CAD build for the part. Positions are in the model's coordinates, mm. Face numbers are marked on the shaded views. A direction names the side the tool comes from. Coordinates: 2 decimals unless noted, no trailing zeros. Order: outer loops, then holes, each group sorted by start corner. A loop starts at its lowest first (then second) coordinate and runs counter-clockwise, first axis right, second up. Notation, with made-up numbers: M -13,89 L 30,89 A25 cw 30,116 Z; hole C -23,71.25 d2. An arc over 180 degrees is marked long. Write item = value, one per line.
from build123d import *

# Parameters (mm, degrees)
AUFSATZ_LINEAR_AUSTRAGEN1_DEPTH = 13
SKIZZE2_W                       = 16
SKIZZE2_H                       = 7
SCHNITT_LINEAR_AUSTRAGEN1_DEPTH = 10
SKIZZE4_R                       = 2.5
SCHNITT_LINEAR_AUSTRAGEN2_DEPTH = 3
SKIZZE5_R                       = 3.5
SKIZZE5_R_2                     = 2
SCHNITT_LINEAR_AUSTRAGEN3_DEPTH = 4
SKIZZE6_R                       = 2.1
SCHNITT_LINEAR_AUSTRAGEN4_DEPTH = 4
SKIZZE7_R                       = 5
SKIZZE7_R_2                     = 3.5
AUFSATZ_LINEAR_AUSTRAGEN2_DEPTH = 0.5
AUFSATZ_LINEAR_START            = 0.5
SKIZZE8_R                       = 5
SKIZZE8_R_2                     = 2.1
AUFSATZ_LINEAR_AUSTRAGEN3_DEPTH = 0.5


with BuildPart() as part:
    # Skizze1 → Aufsatz-Linear austragen1 (new body)
    with BuildSketch(Plane.XY):
        with BuildLine():
            ThreePointArc((5, 0), (3.535533906, 3.535533906), (0, 5))
            Line((0, 5), (0, 2))
            ThreePointArc((0, 2), (1.414213562, 1.414213562), (2, 0))
            ThreePointArc((2, 0), (1.414213562, -1.414213562), (0, -2))
            Line((0, -2), (0, -5))
            ThreePointArc((0, -5), (3.535533906, -3.535533906), (5, 0))
        make_face()
        with BuildLine():
            Line((0, 2), (0, 5))
            ThreePointArc((0, 5), (-5, 0), (0, -5))
            Line((0, -5), (0, -2))
            ThreePointArc((0, -2), (-2, 0), (0, 2))
        make_face()
        with BuildLine():
            Line((20, 5), (0, 5))
            ThreePointArc((0, 5), (3.535533906, 3.535533906), (5, 0))
            ThreePointArc((5, 0), (3.535533906, -3.535533906), (0, -5))
            Line((0, -5), (20, -5))
            Line((20, -5), (20, 5))
        make_face()
    extrude(amount=AUFSATZ_LINEAR_AUSTRAGEN1_DEPTH)

    # Skizze2 → Schnitt-Linear austragen1 (cut)
    with BuildSketch(Plane(origin=(0, 5, 0), x_dir=(1, 0, 0), z_dir=(0, 1, 0))):
        with Locations((12, -6.5)):
            Rectangle(SKIZZE2_W, SKIZZE2_H)
    extrude(amount=-SCHNITT_LINEAR_AUSTRAGEN1_DEPTH, mode=Mode.SUBTRACT)

    # Skizze4 → Schnitt-Linear austragen2 (cut)
    with BuildSketch(Plane.XY.offset(3)):
        with Locations((14, 0)):
            Circle(SKIZZE4_R)
    extrude(amount=-SCHNITT_LINEAR_AUSTRAGEN2_DEPTH, mode=Mode.SUBTRACT)

    # Skizze5 → Schnitt-Linear austragen3 (cut)
    with BuildSketch(Plane(origin=(0, 0, 0), x_dir=(-1, 0, 0), z_dir=(0, 0, -1))):
        Circle(SKIZZE5_R)
        Circle(SKIZZE5_R_2, mode=Mode.SUBTRACT)
    extrude(amount=-SCHNITT_LINEAR_AUSTRAGEN3_DEPTH, mode=Mode.SUBTRACT)

    # Skizze6 → Schnitt-Linear austragen4 (cut)
    with BuildSketch(Plane(origin=(0, 0, 10), x_dir=(-1, 0, 0), z_dir=(0, 0, -1))):
        with Locations((-14, 0)):
            Circle(SKIZZE6_R)
    extrude(amount=-SCHNITT_LINEAR_AUSTRAGEN4_DEPTH, mode=Mode.SUBTRACT)

    # Skizze7 → Aufsatz-Linear austragen2 (add)
    with BuildSketch(Plane.XY.offset(3)):
        with Locations(Location((14, 0, 0), (0, 0, 270))):
            Circle(SKIZZE7_R)
        with Locations((14, 0)):
            Circle(SKIZZE7_R_2, mode=Mode.SUBTRACT)
    extrude(amount=AUFSATZ_LINEAR_AUSTRAGEN2_DEPTH)

    # Skizze8 → Aufsatz-Linear austragen3 (add)
    with BuildSketch(Plane(origin=(0, 0, 10), x_dir=(-1, 0, 0), z_dir=(0, 0, -1)).offset(AUFSATZ_LINEAR_START)):
        with Locations(Location((-14, 0, 0), (0, 0, 270))):
            Circle(SKIZZE8_R)
        with Locations((-14, 0)):
            Circle(SKIZZE8_R_2, mode=Mode.SUBTRACT)
    extrude(amount=-AUFSATZ_LINEAR_AUSTRAGEN3_DEPTH)


solid = part.part
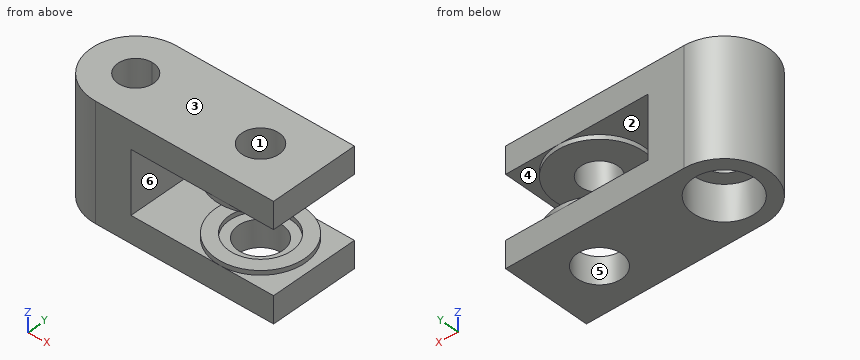
(1) Tool access for the marked faces 4, 5 and 6: list every direction of +Z, -Z, +X, -X, +Y, -Y with a clear straight run to the whole face (end or side of a thin tool).
Evaluation:
face_4 = +X
face_5 = -Z
face_6 = +Y, -Y
(2) Pull direction Z, two halves, no side cores. Call the marked faces 1, 2 and 3: +Z half, -Z half, draft (parallel to the pull), parting line (faces both ways), or undercut.
Evaluation:
face_1 = draft
face_2 = undercut
face_3 = +Z half
(3) Slice it at D-D, the plane y = -3. Write the cut outline in (x, z).
Evaluation:
outline = M -4,0 L -1.8,0 L -1.8,4 L 1.8,4 L 1.8,0 L 20,0 L 20,3 L 18,3 L 18,3.5 L 15.8,3.5 L 15.8,3 L 12.2,3 L 12.2,3.5 L 10,3.5 L 10,3 L 4,3 L 4,10 L 10,10 L 10,9.5 L 18,9.5 L 18,10 L 20,10 L 20,13 L -4,13 Z
(4) Wall check: line 1 (Z direction, x = 16, y = -3); line 2 (Z direction, x = 4.75, y = -0.75); line 3 (Y direction, x = 0, z = 1). Give the ranges that are in metal, low to high. Write a range as from..to.
Evaluation:
line_1 = 0..3.5, 9.5..13
line_2 = 0..3, 10..13
line_3 = -5..-3.5, 3.5..5
(5) Slice it at C-C, the plane z = 11.5. Write the cut outline in (x, y), then the cut area to 3 significant figures.
Evaluation:
outline = M 0,-5 L 20,-5 L 20,5 L 0,5 A5 ccw Z; hole C 0,0 d4; hole C 14,0 d4.2
area = 213 mm²
(6) Slice it at B-B, the plane x = 10.25. Write the cut outline in (y, z).
Evaluation:
outline = M -5,0 L 5,0 L 5,3 L 3.31,3 L 3.31,3.5 L -3.31,3.5 L -3.31,3 L -5,3 Z; M -5,10 L -3.31,10 L -3.31,9.5 L 3.31,9.5 L 3.31,10 L 5,10 L 5,13 L -5,13 Z
(7) Pin check, flat tips, straight feed: pin 1 Ø3 at (x, y) = (10, 1) entering from -Z; pin 2 Ø6 at (y, z) = (-3.5, 6) entering from -X; pin 3 Ø2 at (y, z) = (-1.5, 8) entering from +X. Stop position of each tip, or through.
Evaluation:
pin_1 = 0
pin_2 = -4.97
pin_3 = 4
(8) Slice it at A-A, the plane z = 6. Write the cut outline in (x, y), then the cut area to 3 significant figures.
Evaluation:
outline = M 0,-5 L 4,-5 L 4,5 L 0,5 A5 ccw Z; hole C 0,0 d4
area = 66.7 mm²
